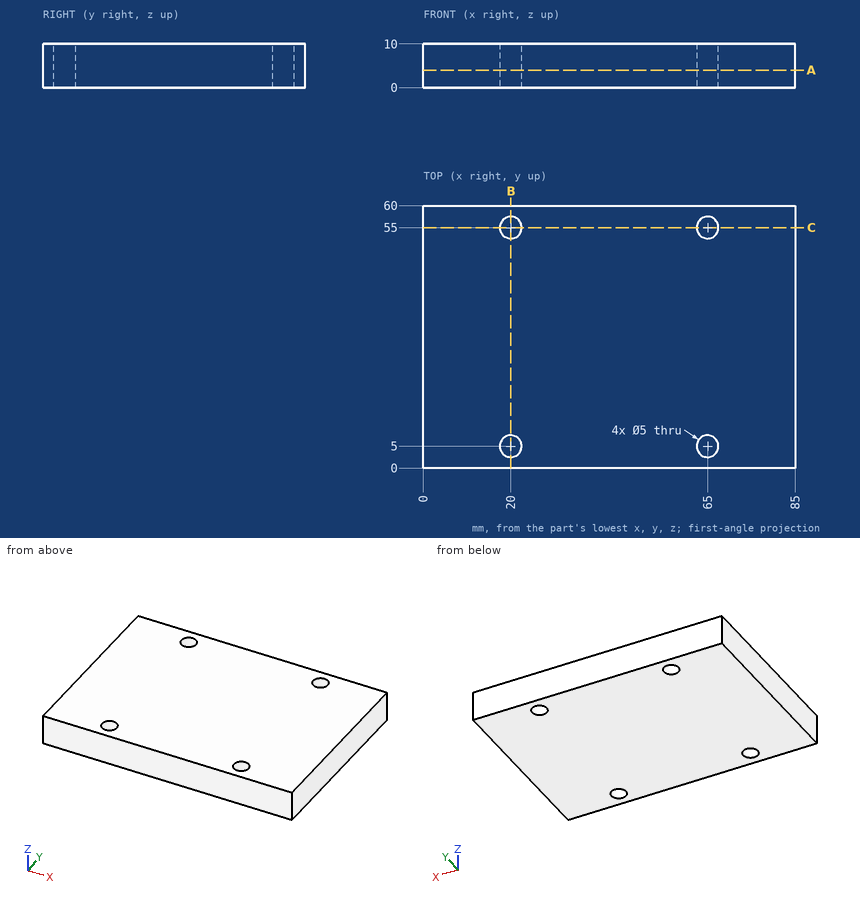
Check sheet for the drawn part. Datum: minimum x, y, z corner. Units: mm. Give positions to 0.01 mm unless a question says otherwise; leave off trailing zeros. Write each loop counter-clockwise with the first axis right and the second up, starting at its lowest first coordinate (ties: lowest second). Pieces come first, ordered by that corner, then holes. Notation, with made-up numbers: M 5,-10.5 L 36,-10.5 A6 ccw 36,0.5 Z; hole C 31,81.5 d10. An arc over 180 degrees is marked long. One line per question, with ' | ' between items.
1. Scan lines: line 1 along X through (y, z) = (55, 1); line 2 along Y through (x, z) = (65, 4.5); line 3 along Y through (x, z) = (22, 7). Record each from-to range of solid material in increasing order. Write a range as from..to.
Ans:
line 1: 0..17.5, 22.5..62.5, 67.5..85 | line 2: 0..2.5, 7.5..52.5, 57.5..60 | line 3: 0..3.5, 6.5..53.5, 56.5..60
2. Cross-section at B-B (x = 20). Enter the section's corners in (y, z), plus the area to 3 significant figures.
Ans:
outline: M 0,0 L 2.5,0 L 2.5,10 L 0,10 Z; M 7.5,0 L 52.5,0 L 52.5,10 L 7.5,10 Z; M 57.5,0 L 60,0 L 60,10 L 57.5,10 Z | area: 500 mm2
3. Cross-section at A-A (z = 4). Enter the section's corners in (x, y), plus the area to 3 significant figures.
Ans:
outline: M 0,0 L 85,0 L 85,60 L 0,60 Z; hole C 20,5 d5; hole C 20,55 d5; hole C 65,5 d5; hole C 65,55 d5 | area: 5,020 mm2
4. Cross-section at C-C (y = 55). Enter the section's corners in (x, z).
Ans:
outline: M 0,0 L 17.5,0 L 17.5,10 L 0,10 Z; M 22.5,0 L 62.5,0 L 62.5,10 L 22.5,10 Z; M 67.5,0 L 85,0 L 85,10 L 67.5,10 Z
